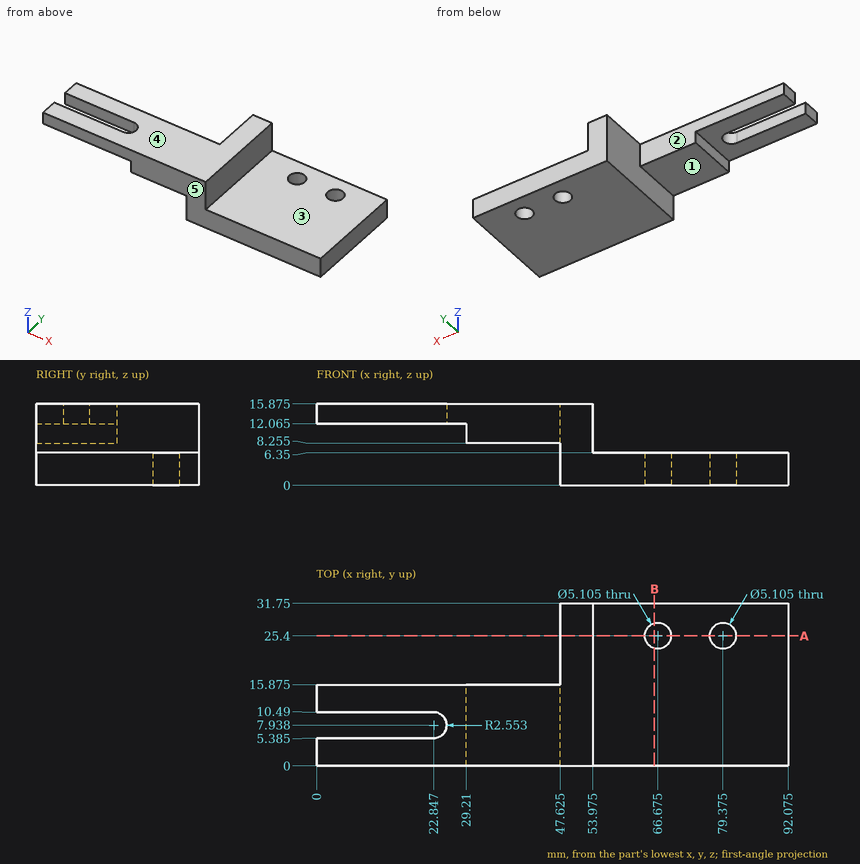
Part print with two shaded views. Sizes in mm from the minimum x, y, z corner. A direction names the side the tool comes from. Coordinates: 2 decimals unless noted, no trailing zeros. Write each loop counter-clockwise with the first axis right and the second up, starting at its lowest first coordinate (ties: lowest second). Pieces come first, ordered by that corner, then holes. Notation, with made-up numbers: (13.5, -5) - (42.5, -5) arc R25 ccw to (42.5, 11) - close; hole circle Ø6 at (17.5, 19.5). An arc over 180 degrees is marked (long way). Put each result on its own line as item: value.
1. Band-saw the part on A-A (y = 25.4). Give the number of separate pieces and of enclosed holes in the cut face, then the cut area to 3 significant figures.
Final values:
separate pieces: 3
enclosed holes: 0
area: 278 mm²
2. Flat gauge pins, fed straight in: pin 1 Ø3 at (y, z) = (22.5, 9.5) entering from +X (1 decimal); pin 2 Ø8 at (y, z) = (21.5, 6) entering from -X (1 decimal); pin 3 Ø3 at (x, z) = (9, 14) entering from -Y; pin 4 Ø5 at (x, y) = (38.5, 14.5) entering from -Z (1 decimal). Where does each tip first touch, or does it go through?
Final values:
pin 1: stops at x = 54
pin 2: stops at x = 47.6
pin 3: stops at y = 0
pin 4: stops at z = 8.3
3. 3-axis set-ups, long thin cutter, end or side, ignore diameter. For the marked faces 1, 2, 3, 4 and 5: which of +Z, -Z, +X, -X, +Y, -Y reach the whole face in a straight line?
Final values:
face 1: -Z, -X, +Y, -Y
face 2: +Z, -Z, -X, +Y
face 3: +Z, +X, +Y, -Y
face 4: +Z, +X, -X, +Y, -Y
face 5: +Z, -Z, +X, -X, -Y
4. Probe line 1 along Y through (x, z) = (40, 12.25) (1 decimal); line 2 along Z through (x, y) = (84.5, 24); line 3 along X through (y, z) = (23.5, 10.75) (1 decimal). List the from-to ranges inside material, lowest first. Write a range as [from, to].
Final values:
line 1: y = [0, 15.9]
line 2: z = [0, 6.35]
line 3: x = [47.6, 54]
5. Band-saw the part on B-B (x = 66). Write the cut outline in (y, z).
Final values:
outline: (0, 0) - (22.94, 0) - (22.94, 6.35) - (0, 6.35) - close; (27.86, 0) - (31.75, 0) - (31.75, 6.35) - (27.86, 6.35) - close
